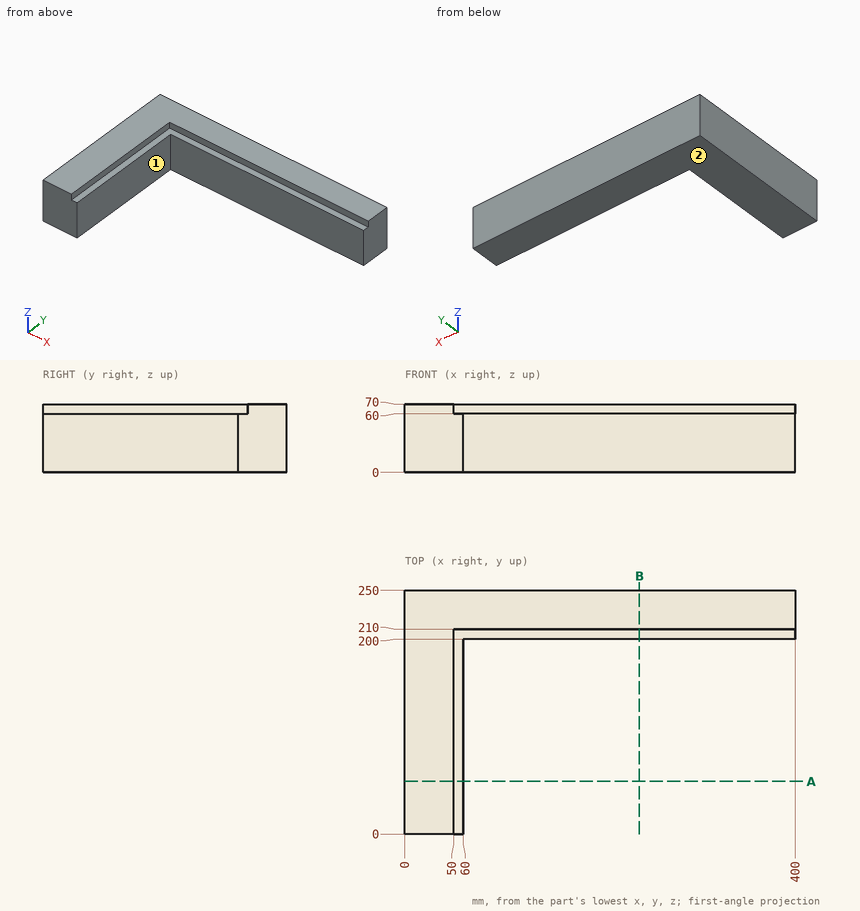
The figure shows three views and two pictorial views of one solid part (mm, origin at its lowest corner). Answer the questions. A direction names the side the tool comes from. Coordinates: 2 decimals unless noted, no trailing zeros. Write each loop counter-clockwise with the first axis right and the second up, starting at its lowest first coordinate (ties: lowest second). Pieces come first, ordered by that corner, then holes.
1. Flat-ended cylindrical pins translate along their axes: pin 1 (11 mm diameter, centred on x = 190, z = 66.5, fed in from -Y); pin 2 (18 mm diameter, centred on y = 57.5, z = 28, fed in from +X); pin 3 (3 mm diameter, centred on y = 156, z = 63.5, fed in from +X). Find the tip coordinate at first contact, or state that the pin passes through.
Results list:
pin 1: stops at y = 210
pin 2: stops at x = 60
pin 3: stops at x = 50
2. The part is cut by section B-B, the plane x = 240.5. Write down the section's boundary in (y, z).
Results list:
outline: (200, 0) - (250, 0) - (250, 70) - (210, 70) - (210, 60) - (200, 60) - close
3. For the marked faces 1 and 2, determine the directions among +Z, -Z, +X, -X, +Y, -Y from which every point of the face is accessible in a straight line to the end or side of a thin tool.
Results list:
face 1: +Z, -Z, +X, -Y
face 2: -Z, +X, -X, +Y, -Y
4. Consider line 1 along X through (y, z) = (196, 11); line 2 along Y through (x, z) = (286, 11.5). Determine where each line is inside the solid, lowest interval first.
Results list:
line 1: x = 0 to 60
line 2: y = 200 to 250
5. The part is cut by section A-A, the plane y = 54. Write down the section's boundary in (x, z).
Results list:
outline: (0, 0) - (60, 0) - (60, 60) - (50, 60) - (50, 70) - (0, 70) - close
